Model file for the job. Use its own axes, mm. Round coordinates to 2 decimals unless told otherwise and drop trailing zeros. Order: outer loops, then holes, each group sorted by start corner. A loop starts at its lowest first (then second) coordinate and runs counter-clockwise, first axis right, second up. Notation, with made-up numbers: (-21, 32.25) - (26, 32.25) arc R18 ccw to (26, 54.25) - close; hole circle Ø3 at (-39, -8.75). An arc over 180 degrees is marked (long way). Answer as CSV lines item,"result". Start each with the question number.
1. Band-saw the part on A-A on z = 0. List the corners of the cut face in (x, y), then the cut area to 3 significant figures.
2. Wall check: line 1 along X through (y, z) = (-0.4, 50); line 2 along Z through (x, y) = (4.5, -1); line 3 along X through (y, z) = (-1.65, -165.5). Give the ranges that are in metal, low to high. Write a range as [from, to].
3. Band-saw the part on C-C on y = -1.7. State how many separate pieces and enclosed holes the cut face has, then the cut area to 3 significant figures.
4. Pin check, flat tips, straight feed: pin 1 Ø1.5 at (x, y) = (-115.5, -1.5) entering from -Z; pin 2 Ø0.9 at (x, y) = (-152.5, -2) entering from -Z; pin 3 Ø1 at (y, z) = (-1, -135) entering from +X. Stop position of each tip, or through.
5. Band-saw the part on B-B on x = 0. List the corners of the cut face in (y, z), then the cut area to 3 significant figures.
6. Band-saw the part on D-D on z = 133. List the corners of the cut face in (x, y).
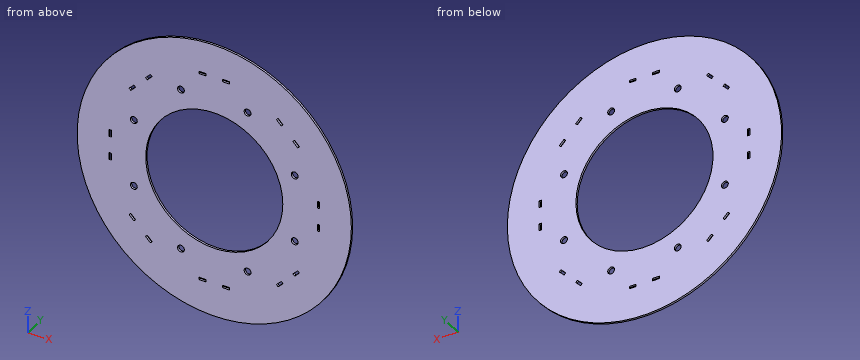
```python
from build123d import *

# Parameters (mm, degrees)
SKETCH_R           = 200
SKETCH_R_2         = 100
SKETCH_W           = 3.25
SKETCH_H           = 10
PAD_DEPTH          = 3
SKETCH001_W        = 3.5
SKETCH001_H        = 10
POCKET_DEPTH       = 1134.38776
POLARPATTERN_COUNT = 8
SKETCH002_R        = 5
POCKET001_DEPTH    = 5


with BuildPart() as part:
    # Sketch → Pad (new body)
    with BuildSketch(Plane.XZ):
        Circle(SKETCH_R)
        Circle(SKETCH_R_2, mode=Mode.SUBTRACT)
        with Locations((-152, 17)):
            Rectangle(SKETCH_W, SKETCH_H, mode=Mode.SUBTRACT)
        with Locations((-152, -17)):
            Rectangle(SKETCH_W, SKETCH_H, mode=Mode.SUBTRACT)
    extrude(amount=PAD_DEPTH)

    # Sketch001 → Pocket (cut, through all)
    with BuildSketch(Plane.XZ):
        with Locations((-152, 17)):
            Rectangle(SKETCH001_W, SKETCH001_H)
        with Locations((-152, -17)):
            Rectangle(SKETCH001_W, SKETCH001_H)
    pocket = extrude(amount=POCKET_DEPTH, mode=Mode.SUBTRACT)

    # PolarPattern: Pocket ×8 about axis
    polarpattern_axis = Axis((0, 0, 0), (0, -1, 0))
    for i in range(1, POLARPATTERN_COUNT):
        add(pocket.rotate(polarpattern_axis, i * 360 / POLARPATTERN_COUNT), mode=Mode.SUBTRACT)

    # Sketch002 → Pocket001 (cut)
    with BuildSketch(Plane.XZ):
        with Locations((-117.332701, 48.600796)):
            Circle(SKETCH002_R)
        with Locations((-48.600796, 117.332701)):
            Circle(SKETCH002_R)
        with Locations((48.600796, 117.332701)):
            Circle(SKETCH002_R)
        with Locations((117.332701, 48.600796)):
            Circle(SKETCH002_R)
        with Locations((117.332701, -48.600796)):
            Circle(SKETCH002_R)
        with Locations((48.600796, -117.332701)):
            Circle(SKETCH002_R)
        with Locations((-48.600796, -117.332701)):
            Circle(SKETCH002_R)
        with Locations((-117.332701, -48.600796)):
            Circle(SKETCH002_R)
    extrude(amount=POCKET001_DEPTH, mode=Mode.SUBTRACT)


solid = part.part
```
Reply:
1,outline,"(-200, -3) - (-100, -3) - (-100, 0) - (-200, 0) - close; (100, -3) - (200, -3) - (200, 0) - (100, 0) - close"
1,area,"600 mm2"
2,line 1,"x = [-193.65, -122.13], [-112.53, -86.6], [86.6, 112.53], [122.13, 193.65]"
2,line 2,"z = [-199.95, -99.9], [99.9, 199.95]"
2,line 3,"x = [-112.29, 112.29]"
3,separate pieces,"1"
3,enclosed holes,"25"
3,area,"93,100 mm2"
4,pin 1,"stops at z = -163.81"
4,pin 2,"stops at z = -129.93"
4,pin 3,"stops at x = 148.02"
5,outline,"(-3, -200) - (0, -200) - (0, -100) - (-3, -100) - close; (-3, 100) - (0, 100) - (0, 200) - (-3, 200) - close"
5,area,"600 mm2"
6,outline,"(-149.37, -3) - (149.37, -3) - (149.37, 0) - (-149.37, 0) - close"
